```python
from build123d import *

# Parameters (mm, degrees)
F0_W     = 60.96
F0_H     = 76.2
F1_DEPTH = 12.7
F2_W     = 5.9436
F2_H     = 76.2
F3_DEPTH = 57.15
F4_W     = 12.7
F4_H     = 76.2
F5_DEPTH = 55.0164
F6_W     = 12.7
F6_H     = 50.8
F7_DEPTH = 63.5
F8_W     = 21.945603
F8_H     = 42.519599
F9_DEPTH = 25.4


with BuildPart() as f1:
    # F0 (on Front) → F1 (new body)
    with BuildSketch(Plane.XZ):
        with Locations((-4.267202, 18.7452)):
            Rectangle(F0_W, F0_H)
    extrude(amount=F1_DEPTH)

    # F2 (on face) → F3 (join)
    with BuildSketch(Plane(origin=(0, 0, 0), x_dir=(-1, 0, 0), z_dir=(0, 1, 0))):
        with Locations((31.775402, 18.7452)):
            Rectangle(F2_W, F2_H)
    extrude(amount=F3_DEPTH)

    # F4 (on face) → F5 (join)
    with BuildSketch(Plane.YZ.offset(-28.803602)):
        with Locations((50.8, 18.7452)):
            Rectangle(F4_W, F4_H)
    extrude(amount=F5_DEPTH)

    # F6 (on face) → F7 (cut)
    with BuildSketch(Plane.YZ.offset(26.212798)):
        with Locations((-6.35, 18.7452)):
            Rectangle(F6_W, F6_H)
    extrude(amount=-F7_DEPTH, mode=Mode.SUBTRACT)

    # F8 (on face) → F9 (cut)
    with BuildSketch(Plane.YZ.offset(-28.803602)):
        with Locations((23.7744, 21.259799)):
            Rectangle(F8_W, F8_H)
    extrude(amount=-F9_DEPTH, mode=Mode.SUBTRACT)


solid = f1.part
```
Geometry: final body of the model. Coordinates: model frame, mm. A direction names the side the tool comes from. Give positions to 0.01 mm unless a question says otherwise; leave off trailing zeros. Order: outer loops, then holes, each group sorted by start corner. A loop starts at its lowest first (then second) coordinate and runs counter-clockwise, first axis right, second up. Notation, with made-up numbers: (28, 47) -> (58, 47) arc R18 ccw to (58, 72) -> close; hole circle Ø2 at (60, -11.75). An arc over 180 degrees is marked (long way). Write each question's results on one line, items separated by ' | '. Start each with the question number.
1) Section B-B (x = -6). Return loops of the section in (y, z), then the cut area to 3 significant figures.
2) Section D-D (y = -8). Return loops of the section in (x, z), then the cut area to 3 significant figures.
3) Section C-C (z = 2.5). Return loops of the section in (x, y), then the cut area to 3 significant figures.
4) Set-up query: faces 5 (the flat face through (-32, 0, 18)), 6 (the flat face through (-32, 24, 42.52)), 7 (the flat face through (-2, 0, -13)). Return all of +Z, -Z, +X, -X, +Y, -Y with unobstructed straight access to the full face (end or side cutting, diameter ignored); none if empty.
5) Line query: line 1 (Y direction, x = 6, z = 50.5); line 2 (Y direction, x = 15.5, z = 31.5); line 3 (X direction, y = 36, z = 2). Output: solid intervals per line, ascending. Write a range as from..to.
6) Draft query along Z for faces 1 (the flat face through (26.213, 51, 19)), 2 (the flat face through (-5, 45, 56.845)), 3 (the flat face through (-4, -6, 44.145)), 4 (the flat face through (-32, 34.747, 21)). Return one class per face: pulls with the +Z half, pulls with the -Z half, needs draft (parallel to the pull), parting line crosses it, or undercut.
7) Section A-A (y = 29.5). Return loops of the section in (x, z), then the cut area to 3 significant figures.
8) First-contact query: pin 1 (4 mm diameter, centred on y = 41, z = -6.5, fed in from +X); pin 2 (6.5 mm diameter, centred on x = -32.5, z = 26.5, fed in from -Y); pin 3 (16.5 mm diameter, centred on x = 10, z = 30, fed in from -Y). Flat tips, straight axial feed; report the tip coordinate or a pass-through.
Calculated:
1) outline: (-12.7, -19.35) -> (0, -19.35) -> (0, -6.65) -> (-12.7, -6.65) -> close; (-12.7, 44.15) -> (0, 44.15) -> (0, 56.85) -> (-12.7, 56.85) -> close; (44.45, -19.35) -> (57.15, -19.35) -> (57.15, 56.85) -> (44.45, 56.85) -> close | area: 1,290 mm2
2) outline: (-34.75, -19.35) -> (26.21, -19.35) -> (26.21, -6.65) -> (-34.75, -6.65) -> close; (-34.75, 44.15) -> (26.21, 44.15) -> (26.21, 56.85) -> (-34.75, 56.85) -> close | area: 1,550 mm2
3) outline: (-34.75, 0) -> (-28.8, 0) -> (-28.8, 12.8) -> (-34.75, 12.8) -> close; (-34.75, 34.75) -> (-28.8, 34.75) -> (-28.8, 44.45) -> (26.21, 44.45) -> (26.21, 57.15) -> (-34.75, 57.15) -> close | area: 908 mm2
4) face 5: +X, -X, -Y | face 6: +X, -X | face 7: +Z, -Z, +X
5) line 1: -12.7..0, 44.45..57.15 | line 2: 44.45..57.15 | line 3: -34.75..-28.8
6) face 1: needs draft | face 2: pulls with the +Z half | face 3: undercut | face 4: undercut
7) outline: (-34.75, -19.35) -> (-28.8, -19.35) -> (-28.8, 0) -> (-34.75, 0) -> close; (-34.75, 42.52) -> (-28.8, 42.52) -> (-28.8, 56.85) -> (-34.75, 56.85) -> close | area: 200 mm2
8) pin 1: x = -28.8 | pin 2: y = 0 | pin 3: y = 44.45
